Autodesk Inventor part; units mm, degrees
ref_plane "Work Plane1" through (41.411, -174.5481, 0) normal (0, -1, 0) x (1, 0, 0)
ref_plane "YZ Plane" through (0, 0, 0) normal (1, 0, 0) x (0, 1, 0)
ref_plane "XZ Plane" through (0, 0, 0) normal (0, 1, 0) x (-1, 0, 0)
sketch "Sketch1" plane through (0, 0, 0) normal (0, 0, 1) x (1, 0, 0)
  line L0 (0, 0) -> (160, 0) construction
  line L1 (160, 0) -> (118.589, -154.5481) construction
  line L2 (0, 0) -> (41.411, -154.5481) construction
  line L3 (41.411, -154.5481) -> (118.589, -154.5481)
  circle A0 centre (235.8871, -103.156) radius 80 construction
  line L4 (160, 0) -> (256.5926, -25.8819)
  line L5 (118.589, -154.5481) -> (215.1815, -180.43)
  arc A1 (215.1815, -180.43) -> (256.5926, -25.8819) centre (235.8871, -103.156) ccw
  circle A2 centre (-75.8871, -103.156) radius 80 construction
  line L6 (0, 0) -> (-96.5926, -25.8819)
  line L7 (41.411, -154.5481) -> (-55.1815, -180.43)
  arc A3 (-96.5926, -25.8819) -> (-55.1815, -180.43) centre (-75.8871, -103.156) ccw
  arc A4 (160, 0) -> (0, 0) centre (80, -304.672) ccw
  dimension "d0" = 160
  dimension "d1" = 160
  dimension "d2" = 160
  dimension "d3" = 75
  dimension "d4" = 75
  dimension "d5" = 160
  dimension "d6" = 100
  dimension "d7" = 160
  dimension "d9" = 100
  dimension "d56" = 315
extrude "Extrusion1" add sketch "Sketch1" along normal blind 41.5
sketch "Sketch2" plane through (0, 0, 41.5) normal (0, 0, 1) x (1, 0, 0)
  line L0 (-26.5, -133) -> (186.5, -133)
  line L1 (186.5, -133) -> (186.5, -20)
  line L2 (186.5, -20) -> (-26.5, -20)
  line L3 (-26.5, -20) -> (-26.5, -133)
  line L4 (0, 0) -> (-96.5926, -25.8819)
  arc A0 (160, 0) -> (0, 0) centre (80, -304.672) ccw
  line L5 (0, 0) -> (160, 0)
  point P0 (80, -20)
  point P1 (80, 0)
  dimension "d12" = 213
  dimension "d13" = 113
  dimension "d57" = 20
extrude "Extrusion2" cut sketch "Sketch2" against normal through all contours L3 L2 L1 L0
sketch "Sketch3" plane through (0, 0, 41.5) normal (0, 0, 1) x (1, 0, 0)
  line L0 (186.5, -20) -> (186.5, -133) construction
  line L1 (186.5, -133) -> (-26.5, -133) construction
  line L2 (-26.5, -133) -> (-26.5, -20) construction
  line L3 (-26.5, -20) -> (186.5, -20) construction
  line L4 (0, 0) -> (-96.5926, -25.8819) construction
  arc A0 (-96.5926, -25.8819) -> (-55.1815, -180.43) centre (-75.8871, -103.156) ccw construction
  line L5 (-55.1815, -180.43) -> (41.411, -154.5481) construction
  line L6 (41.411, -154.5481) -> (118.589, -154.5481) construction
  line L7 (118.589, -154.5481) -> (215.1815, -180.43) construction
  arc A1 (215.1815, -180.43) -> (256.5926, -25.8819) centre (235.8871, -103.156) ccw construction
  line L8 (256.5926, -25.8819) -> (160, 0) construction
  line L9 (-48.0481, -154.5481) -> (208.0481, -154.5481) construction
  line L10 (208.0481, -154.5481) -> (208.0481, 10.328) construction
  line L11 (-48.0481, 10.328) -> (-48.0481, -154.5481) construction
  line L12 (-48.0481, 10.328) -> (-48.0481, -178.5186)
  line L13 (-55.1815, -180.43) -> (41.411, -154.5481)
  line L14 (208.0481, 10.328) -> (208.0481, -178.5186)
  line L15 (118.589, -154.5481) -> (215.1815, -180.43)
  line L16 (-48.0481, -178.5186) -> (208.0481, -178.5186)
  line L17 (-48.0481, 10.328) -> (208.0481, 10.328)
  line L18 (-157.6505, -218.8456) -> (317.6505, -218.8456)
  line L19 (317.6505, -218.8456) -> (317.6505, 50.655)
  line L20 (317.6505, 50.655) -> (-157.6505, 50.655)
  line L21 (-157.6505, 50.655) -> (-157.6505, -218.8456)
  arc A2 (160, 0) -> (0, 0) centre (80, -304.672) ccw
  point P0 (80, -154.5481)
  point P1 (80, 10.328)
  point P2 (208.0481, -84.0953)
  point P3 (317.6505, -84.0953)
  point P4 (80, 10.328)
  point P5 (80, -218.8456)
  dimension "d22" = 269.5006
  dimension "d23" = 475.3011
extrude "Extrusion3" cut sketch "Sketch3" against normal through all
sketch "Sketch5" plane through (0, 0, 41.5) normal (0, 0, 1) x (1, 0, 0)
  line L0 (118.589, -154.5481) -> (208.0481, -178.5186)
  line L1 (208.0481, -178.5186) -> (80, -178.5186)
  line L2 (80, -178.5186) -> (80, 10.328)
  line L3 (80, 10.328) -> (208.0481, 10.328)
  line L4 (208.0481, 10.328) -> (208.0481, -178.5186)
  arc A0 (160, 0) -> (0, 0) centre (80, -304.672) ccw
extrude "Extrusion4" cut sketch "Sketch5" against normal through all
sketch "Sketch6" plane through (0, 0, 0) normal (0, 1, 0) x (-1, 0, 0)
  circle A0 centre (17, 20.75) radius 2
  line L0 (26.5, 41.5) -> (26.5, 0)
  point P0 (26.5, 20.75)
  dimension "d24" = 4
  dimension "d58" = 9.5
extrude "Extrusion5" cut sketch "Sketch6" along normal through all both and the other way through all
sketch "Sketch7" plane through (0, 0, 0) normal (0, 1, 0) x (-1, 0, 0)
  circle A0 centre (17, 20.75) radius 2
  circle A1 centre (17, 20.75) radius 6.5
  dimension "d59" = 13
extrude "Extrusion6" cut sketch "Sketch7" against normal blind 10
ref_plane "Work Plane1" through (41.411, -174.5481, 0) normal (0, -1, 0) x (1, 0, 0)
sketch "Sketch8" plane through (41.411, -174.5481, 0) normal (0, -1, 0) x (1, 0, 0)
  circle A0 centre (-58.411, 20.75) radius 2
  circle A1 centre (-58.411, 20.75) radius 6.5
  point P0 (-41.411, 0)
  dimension "d32" = 13
extrude "Extrusion7" cut sketch "Sketch8" against normal blind 10
sketch "Sketch11" plane through (41.411, -154.5481, 0) normal (0, -1, 0) x (1, 0, 0)
  line L0 (0, 41.5) -> (38.589, 41.5)
  line L1 (0, 0) -> (0, 41.5)
  line L2 (0, 0) -> (38.589, 0)
  line L3 (38.589, 0) -> (38.589, 41.5)
  circle A0 centre (19.2945, 20.75) radius 2.5
  circle A1 centre (19.2945, 20.75) radius 6.5
  point P0 (-41.411, 0)
  point P1 (0, 20.75)
  point P2 (19.2945, 41.5)
  dimension "d73" = 5
  dimension "d74" = 13
extrude "Extrusion10" cut sketch "Sketch11" against normal blind 10 contours A1
sketch "Sketch12" plane through (-48.0481, -178.5186, 41.5) normal (-1, 0, 0) x (0, 0, 1)
  line L0 (-41.5, 0) -> (-41.5, 165.6442)
  line L1 (0, 0) -> (-41.5, 0)
  line L2 (0, 165.6442) -> (0, 0)
  line L3 (-41.5, 165.6442) -> (0, 165.6442)
  line L4 (-5, 5) -> (-36.5, 5)
  line L5 (-36.5, 5) -> (-36.5, 160.6442)
  line L6 (-36.5, 160.6442) -> (-5, 160.6442)
  line L7 (-5, 160.6442) -> (-5, 5)
  point P0 (-41.5, 178.5186)
  dimension "d43" = 5
extrude "Extrusion11" cut sketch "Sketch12" against normal blind 15 contours L4 L5 L6 L7
sketch "Sketch13" plane through (0, 0, 41.5) normal (0, 0, 1) x (1, 0, 0)
  circle A0 centre (-40.0481, -95.6966) radius 2.5
  line L0 (-48.0481, -12.8745) -> (-48.0481, -178.5186)
  point P0 (0, 0)
  point P1 (-48.0481, -95.6966)
  dimension "d46" = 5
  dimension "d47" = 8
extrude "Extrusion12" cut sketch "Sketch13" against normal through all
sketch "Sketch14" plane through (0, 0, 41.5) normal (0, 0, 1) x (1, 0, 0)
  circle A0 centre (-40.0481, -95.6966) radius 2.5
  circle A1 centre (-40.0481, -95.6966) radius 6.5
  point P0 (0, 0)
  dimension "d50" = 13
extrude "Extrusion13" cut sketch "Sketch14" against normal blind 4
sketch "Sketch15" plane through (0, 0, 0) normal (0, 0, -1) x (-1, 0, 0)
  circle A0 centre (40.0481, -95.6966) radius 2.5
  circle A1 centre (40.0481, -95.6966) radius 2.5
  circle A2 centre (40.0481, -95.6966) radius 6.5
  point P0 (0, 0)
  dimension "d53" = 13
extrude "Extrusion14" cut sketch "Sketch15" against normal blind 4
sketch "Sketch16" plane through (0, 0, 41.5) normal (0, 0, 1) x (1, 0, 0)
  line L0 (80, -20) -> (80, 10.328) construction
  circle A0 centre (80, -4.836) radius 7 construction
  circle A1 centre (80, -4.836) radius 15.164 construction
  arc A2 (80, -20) -> (80, 10.328) centre (80, -4.836) ccw
  arc A3 (80, -11.836) -> (80, 2.164) centre (80, -4.836) ccw
  arc A4 (80, 10.328) -> (0, 0) centre (80, -304.672) ccw
  line L1 (80, 10.328) -> (80, 2.164)
  line L2 (80, -11.836) -> (80, -20)
  dimension "d62" = 14
extrude "Extrusion15" add sketch "Sketch16" against normal blind 41.5
sketch "Sketch17" plane through (0, 0, 41.5) normal (0, 0, 1) x (1, 0, 0)
  arc A0 (80, -11.836) -> (80, 2.164) centre (80, -4.836) ccw construction
  circle A1 centre (80, -4.836) radius 7
  point P0 (0, 0)
extrude "Extrusion16" cut sketch "Sketch17" against normal through all
sketch "Sketch19" plane through (0, 0, 41.5) normal (0, 0, 1) x (1, 0, 0)
  circle A0 centre (80, -4.836) radius 7
  arc A1 (80, -20) -> (80, 10.328) centre (80, -4.836) ccw
  circle A2 centre (80, -4.836) radius 15.164 construction
  circle A3 centre (80, -4.836) radius 16.164
  point P0 (0, 0)
  dimension "d72" = 1
extrude "Extrusion18" cut sketch "Sketch19" against normal blind 20.75
sketch "Sketch20" plane through (60.7055, -154.5481, 20.75) normal (0, -1, 0) x (1, 0, 0)
  circle A0 centre (0, 0) radius 2.5
  point P0 (-60.7055, -20.75)
extrude "Extrusion19" cut sketch "Sketch20" against normal blind 50
sketch "Sketch21" plane through (0, 0, 20.75) normal (0, 0, 1) x (1, 0, 0)
  circle A0 centre (80, -4.836) radius 6.5
  circle A1 centre (80, -4.836) radius 10
  point P0 (0, 0)
  dimension "d77" = 20
extrude "Extrusion20" cut sketch "Sketch21" against normal blind 15.5 contours A0 | A1
properties part number "Riser Base" material "ABS Plastic"
Could you check a few things on this model? Use its own coordinates, in mm. A direction names the side the tool comes from. Give positions to 0.01 mm unless a question says otherwise; leave off trailing zeros. Order: outer loops, then holes, each group sorted by start corner. A loop starts at its lowest first (then second) coordinate and runs counter-clockwise, first axis right, second up. Notation, with made-up numbers: M 71,76.25 L 116,76.25 A23 ccw 116,96.25 Z; hole C 39.25,86.5 d9. An arc over 180 degrees is marked long. One line per question, with ' | ' between items.
1. I want a section at A-A (y = -152). List the corners of the cut face in (x, z) for me.
Results:
outline: M -48.05,0 L 80,0 L 80,41.5 L -48.05,41.5 L -48.05,36.5 L -33.05,36.5 L -33.05,5 L -48.05,5 Z; hole C -17,20.75 d4; hole C 60.71,20.75 d13
2. If I drill on line 1 (Z direction, x = -17, y = -16.75); line 2 (Y direction, x = 72, z = 38.5); line 3 (Y direction, x = 70, z = 21.5), over which ranges is the centre line in solid material (lowest first)?
Results:
line 1: 0 to 18.75, 22.75 to 41.5 | line 2: -154.55 to -133, -20 to -18.88, 9.21 to 10.23 | line 3: -154.55 to -133, -20 to -17.54, 7.86 to 10.17
3. I'm going to push flat-ended pins straight in: pin 1 (6.5 mm diameter, centred on x = -15, z = 22.5, fed in from -Y); pin 2 (16 mm diameter, centred on x = 80, y = -4.836, fed in from +Z); pin 3 (3 mm diameter, centred on y = -141.5, z = 36.5, fed in from +X); pin 4 (3.5 mm diameter, centred on x = -17, z = 20.75, fed in from -Y). Where does each tip first touch, or does it pass through?
Results:
pin 1: y = -164.55 | pin 2: z = 5.25 | pin 3: x = 80 | pin 4: through
4. I want a section at D-D (y = -69.5). List the corners of the cut face in (x, z) for me, and give its area (3 significant figures).
Results:
outline: M -48.05,0 L -26.5,0 L -26.5,41.5 L -48.05,41.5 L -48.05,36.5 L -33.05,36.5 L -33.05,5 L -48.05,5 Z | area: 422 mm²
5. I want a section at C-C (x = -17). List the corners of the cut face in (y, z) for me.
Results:
outline: M -170.2,0 L -133,0 L -133,18.75 L -164.55,18.75 L -164.55,14.25 L -170.2,14.25 Z; M -170.2,27.25 L -164.55,27.25 L -164.55,22.75 L -133,22.75 L -133,41.5 L -170.2,41.5 Z; M -20,0 L -4.56,0 L -4.56,14.25 L -10,14.25 L -10,18.75 L -20,18.75 Z; M -20,22.75 L -10,22.75 L -10,27.25 L -4.56,27.25 L -4.56,41.5 L -20,41.5 Z
6. I want a section at B-B (x = 35.5). List the corners of the cut face in (y, z) for me.
Results:
outline: M -156.13,0 L -133,0 L -133,41.5 L -156.13,41.5 Z; M -20,0 L 7.17,0 L 7.17,41.5 L -20,41.5 Z
7. For faces 1 (the face through (61, -144.548, 18)), 2 (the face through (70.01, -4.4, 13.11)), 3 (the face through (27, -20, 21)), 4 (the face through (56, -154.548, 16)), which set-ups out of +Z, -Z, +X, -X, +Y, -Y let a thin tool reach every point of the face, with its end or its side?
Results:
face 1: -Y | face 2: +Z | face 3: +Z, -Z, +X | face 4: +Z, -Z, +X, -Y
8. We'd pull the mould along X, two halves only. Please class faces 5 (the face through (-15.526, -148.553, 22.102)), 6 (the face through (-28, -83, 41.5)), 7 (the face through (-10.506, -7.145, 21.036)), 8 (the face through (95.16, -5.17, 10.52)): +X half, -X half, draft (parallel to the pull), parting line (faces both ways), or undercut.
Results:
face 5: undercut | face 6: draft | face 7: undercut | face 8: +X half
